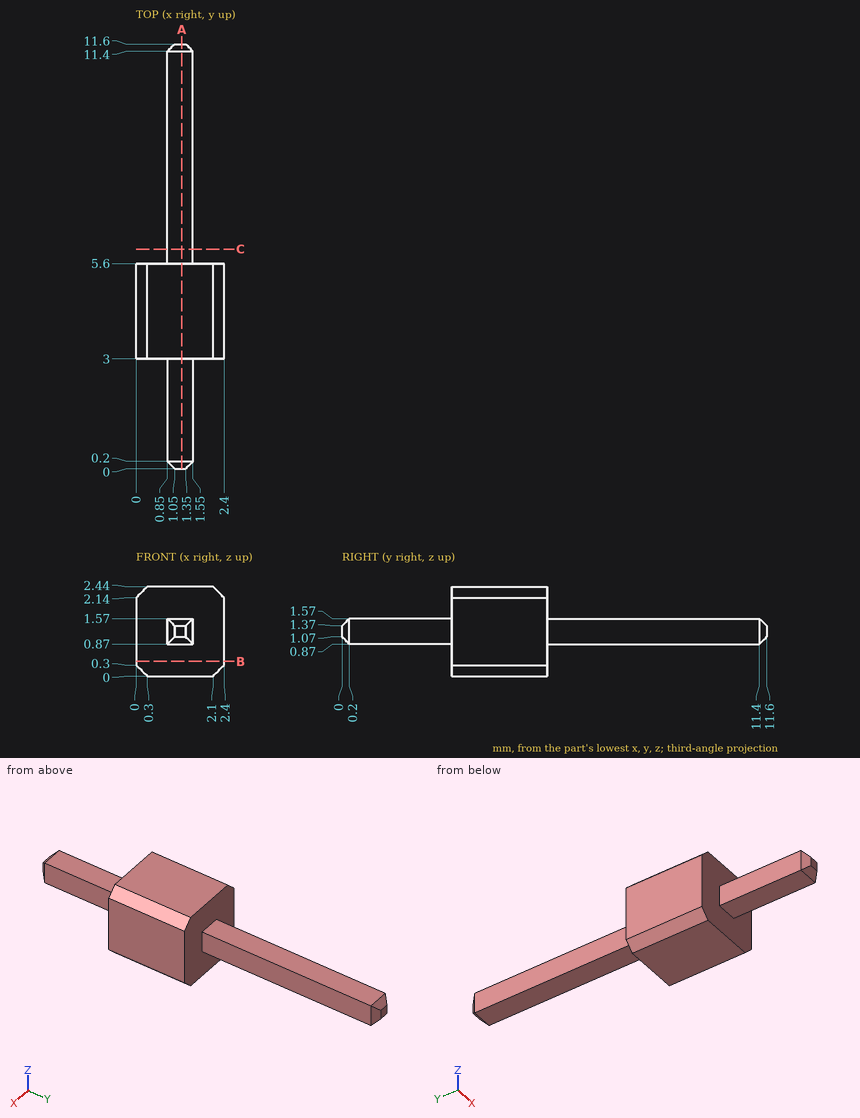
Input: dimensioned drawing with shaded views. Units: mm. Origin: part minimum x, y, z. Round coordinates to 2 decimals unless told otherwise and drop trailing zeros. Order: outer loops, then holes, each group sorted by start corner. A loop starts at its lowest first (then second) coordinate and runs counter-clockwise, first axis right, second up.
1. Cut plane A-A, the plane x = 1.25. Output: boundary loops of the cut face in (y, z), then the cut area to 3 significant figures.
The answers:
outline: (0, 1.07) - (0.2, 0.87) - (3, 0.87) - (3, 0) - (5.6, 0) - (5.6, 0.87) - (11.4, 0.87) - (11.6, 1.07) - (11.6, 1.37) - (11.4, 1.57) - (5.6, 1.57) - (5.6, 2.44) - (3, 2.44) - (3, 1.57) - (0.2, 1.57) - (0, 1.37) - close
area: 12.6 mm2
2. Cut plane C-C, the plane y = 6. Output: boundary loops of the cut face in (x, z), then the cut area to 3 significant figures.
The answers:
outline: (0.85, 0.87) - (1.55, 0.87) - (1.55, 1.57) - (0.85, 1.57) - close
area: 0.490 mm2
3. Cut plane B-B, the plane z = 0.4. Output: boundary loops of the cut face in (x, y).
The answers:
outline: (0, 3) - (2.4, 3) - (2.4, 5.6) - (0, 5.6) - close
4. Pin query (flat end, axial travel): P1, Ø0.8, axis at y = 2, z = 1.5, coming from the +X side; P2, Ø0.6, axis at x = 1, y = 2, coming from the -Z side. Return the tip coordinate at first contact, or that it passes through.
The answers:
P1: stops at x = 1.55
P2: stops at z = 0.87
5. Material intervals for line 1 (Z direction, x = 1.2, y = 10); line 2 (Y direction, x = 0.4, z = 0.85), sorted ascending.
The answers:
line 1: z = 0.87 to 1.57
line 2: y = 3 to 5.6
